Could you check a few things on this drawing? It's one solid part, dimensions in mm from its lowest x, y, z. Round coordinates to 2 decimals unless told otherwise and drop trailing zeros. Loops run counter-clockwise (first coordinate to the right, second up) from the corner with the lowest first, then second, coordinate; pieces in that order, holes last. Notation, with made-up numbers: M 30,88.5 L 53,88.5 A12 ccw 53,100.5 Z; hole C 0,86 d9. An arc over 180 degrees is marked long. Answer as CSV lines item,"result".
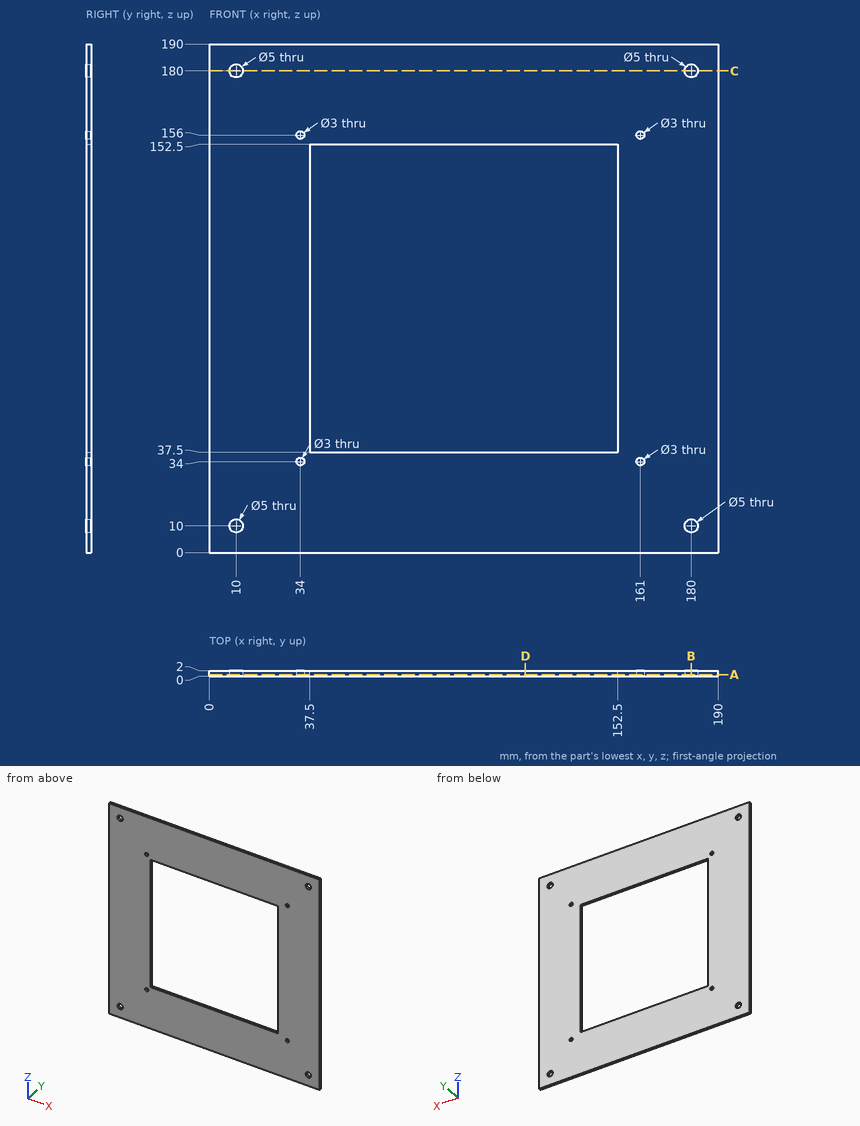
Item 1: If I drill on line 1 along Z through (x, y) = (34, 1.2); line 2 along X through (y, z) = (1.3, 156); line 3 along X through (y, z) = (0.8, 10), over which ranges is the centre line in solid material (lowest first)? Write a range as from..to.
Output:
line 1,"z = 0..32.5, 35.5..154.5, 157.5..190"
line 2,"x = 0..32.5, 35.5..159.5, 162.5..190"
line 3,"x = 0..7.5, 12.5..177.5, 182.5..190"
Item 2: If we section it at B-B on x = 180: Write out the boundary of the cut face in (y, z), then the cut area to 3 significant figures.
Output:
outline,"M 0,0 L 2,0 L 2,7.5 L 0,7.5 Z; M 0,12.5 L 2,12.5 L 2,177.5 L 0,177.5 Z; M 0,182.5 L 2,182.5 L 2,190 L 0,190 Z"
area,"360 mm2"
Item 3: If we section it at C-C on z = 180: Write out the boundary of the cut face in (x, y), then the cut area to 3 significant figures.
Output:
outline,"M 0,0 L 7.5,0 L 7.5,2 L 0,2 Z; M 12.5,0 L 177.5,0 L 177.5,2 L 12.5,2 Z; M 182.5,0 L 190,0 L 190,2 L 182.5,2 Z"
area,"360 mm2"
Item 4: If we section it at D-D on x = 118: Write out the boundary of the cut face in (y, z), then the cut area to 3 significant figures.
Output:
outline,"M 0,0 L 2,0 L 2,37.5 L 0,37.5 Z; M 0,152.5 L 2,152.5 L 2,190 L 0,190 Z"
area,"150 mm2"
Item 5: If we section it at A-A on y = 0.55: State how many separate pieces and enclosed holes the cut face has, then the cut area to 3 significant figures.
Output:
separate pieces,"1"
enclosed holes,"9"
area,"22,800 mm2"
